Part model, mm, in its own coordinate system. A direction names the side the tool comes from. Round coordinates to 2 decimals unless told otherwise and drop trailing zeros. Write each loop counter-clockwise with the first axis right and the second up, starting at its lowest first coordinate (ties: lowest second). Pieces come first, ordered by that corner, then holes. Notation, with made-up numbers: (41, -22) -> (48, -22) arc R12 ccw to (48, -2) -> close; hole circle Ø2 at (-15, 68). An arc over 180 degrees is marked (long way). Return JSON: item names as keys, results as strings. Group by question number.
(1) Mould opens along Z. For faces 1 (the cylindrical face through (-3, 31, 0)), 2 (the flat face through (0.4, -5, 0)), 3 (the cylindrical face through (-1.5, 30.93, 0.07)) say: +Z half, -Z half, draft (parallel to the pull), parting line (faces both ways), or undercut.
(2) Drill centre lines: L1, parallel to Z at x = 0, y = 55.5; L2, parallel to Z at x = 0, y = -4.45; L3, parallel to X at y = 56, z = 1. Where is each one in solid material? Low to high. Write a range as from..to.
(3) Saw through at A-A (y = 43). List the corners of the cut face in (x, z), plus the area to 3 significant figures.
(4) Tool access for faces 4 (the cylindrical face through (-0.217, -4.507, -0.976)), 5 (the flat face through (-1.3, 61, -1.3)): list every direction of +Z, -Z, +X, -X, +Y, -Y with a clear straight run to the whole face (end or side of a thin tool).
(5) Drop flat-ended pins along their axis: pin 1 Ø2 at (y, z) = (31.5, -2.5) entering from -X; pin 2 Ø2 at (x, z) = (1, 0) entering from +Y. Give the stop position or say it passes through.
from build123d import *


with BuildPart() as part:
    # Sketch1 → Revolve1 (revolve)
    with BuildSketch(Plane.XY):
        with BuildLine():
            Line((1.5, 61), (3, 61))
            Line((3, 61), (3, 1))
            add(Edge.make_bspline(
                [(1, -4), (1, -2.852326224), (1, -1.704652447), (3, -1.295347553), (3, -0.147673776), (3, 1)],
                knots=[0, 0, 0, 0, 0, 0, 1, 1, 1, 1, 1, 1], degree=5))
            Line((1, -4), (1, -5))
            Line((1, -5), (0.25, -5))
            Line((0.25, -5), (0.25, -4))
            add(Edge.make_bspline(
                [(0.25, -4), (0.25, -2.870146948), (0.25, -1.740293897), (1.5, -2.259706103), (1.5, -1.129853052), (1.5, 0)],
                knots=[0, 0, 0, 0, 0, 0, 1, 1, 1, 1, 1, 1], degree=5))
            Line((1.5, 0), (1.5, 61))
        make_face()
    revolve(axis=Axis((0, 0, 0), (0, -1, 0)))


solid = part.part
Computed values:
{
 "1": {"face 1": "parting line", "face 2": "draft", "face 3": "undercut"},
 "2": {"L1": "-3..-1.5, 1.5..3", "L2": "-1..-0.25, 0.25..1", "L3": "-2.83..-1.12, 1.12..2.83"},
 "3": {"outline": "circle Ø6 at (0, 0); hole circle Ø3 at (0, 0)", "area": "21.2 mm2"},
 "4": {"face 4": "-Y", "face 5": "+Z, -Z, +X, -X, +Y"},
 "5": {"pin 1": "x = -2.6", "pin 2": "y = 61"}
}
